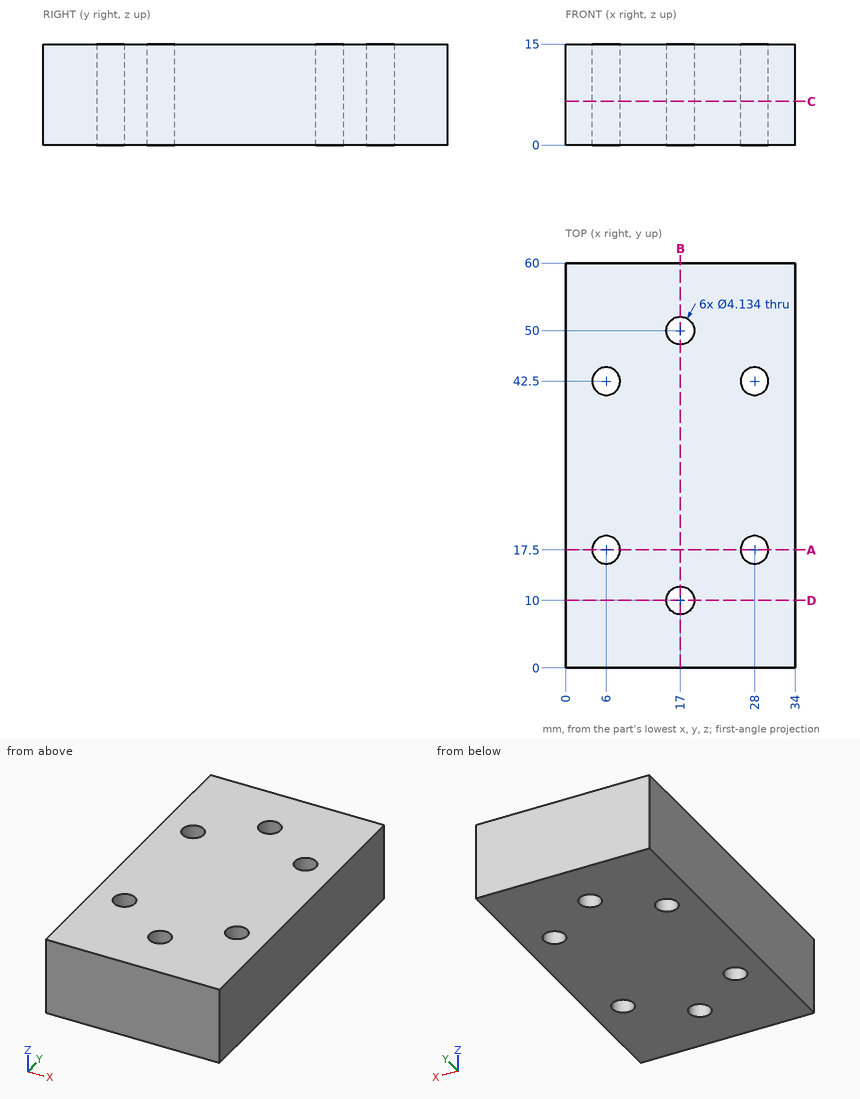
Verification items for this drawing (mm, ordinates from the low corner). Give positions to 0.01 mm unless a question says otherwise; leave off trailing zeros. Write each loop counter-clockwise with the first axis right and the second up, starting at its lowest first coordinate (ties: lowest second). Pieces come first, ordered by that corner, then holes. Notation, with made-up numbers: (26.5, -21.75) -> (42.5, -21.75) arc R21 cw to (42.5, -2.75) -> close; hole circle Ø4 at (3.5, -20). An arc over 180 degrees is marked (long way). Use CSV: the item, a comma, the result in double quotes.
(1) Sectioned sample at C-C (z = 6.5). Record the cut outline in (x, y), plus the area to 3 significant figures.
Derived:
outline,"(0, 0) -> (34, 0) -> (34, 60) -> (0, 60) -> close; hole circle Ø4.13 at (6, 17.5); hole circle Ø4.13 at (6, 42.5); hole circle Ø4.13 at (17, 10); hole circle Ø4.13 at (17, 50); hole circle Ø4.13 at (28, 17.5); hole circle Ø4.13 at (28, 42.5)"
area,"1,960 mm^2"
(2) Sectioned sample at D-D (y = 10). Record the cut outline in (x, z).
Derived:
outline,"(0, 0) -> (14.93, 0) -> (14.93, 15) -> (0, 15) -> close; (19.07, 0) -> (34, 0) -> (34, 15) -> (19.07, 15) -> close"
(3) Material ranges on L1, parallel to Y at x = 6, z = 6; L2, parallel to X at y = 17.5, z = 9.75; L3, parallel to Y at x = 17, z = 9.75, recorded low to high.
Derived:
L1,"y = 0 to 15.43, 19.57 to 40.43, 44.57 to 60"
L2,"x = 0 to 3.93, 8.07 to 25.93, 30.07 to 34"
L3,"y = 0 to 7.93, 12.07 to 47.93, 52.07 to 60"
(4) Sectioned sample at B-B (x = 17). Record the cut outline in (y, z).
Derived:
outline,"(0, 0) -> (7.93, 0) -> (7.93, 15) -> (0, 15) -> close; (12.07, 0) -> (47.93, 0) -> (47.93, 15) -> (12.07, 15) -> close; (52.07, 0) -> (60, 0) -> (60, 15) -> (52.07, 15) -> close"
(5) Go/stop test with a flat-tipped pin: pin 1 (3.5 mm diameter, centred on x = 17, y = 10, fed in from -Z). Record where the tip stops, or that it passes through.
Derived:
pin 1,"passes through"
(6) Sectioned sample at A-A (y = 17.5). Record the cut outline in (x, z).
Derived:
outline,"(0, 0) -> (3.93, 0) -> (3.93, 15) -> (0, 15) -> close; (8.07, 0) -> (25.93, 0) -> (25.93, 15) -> (8.07, 15) -> close; (30.07, 0) -> (34, 0) -> (34, 15) -> (30.07, 15) -> close"
